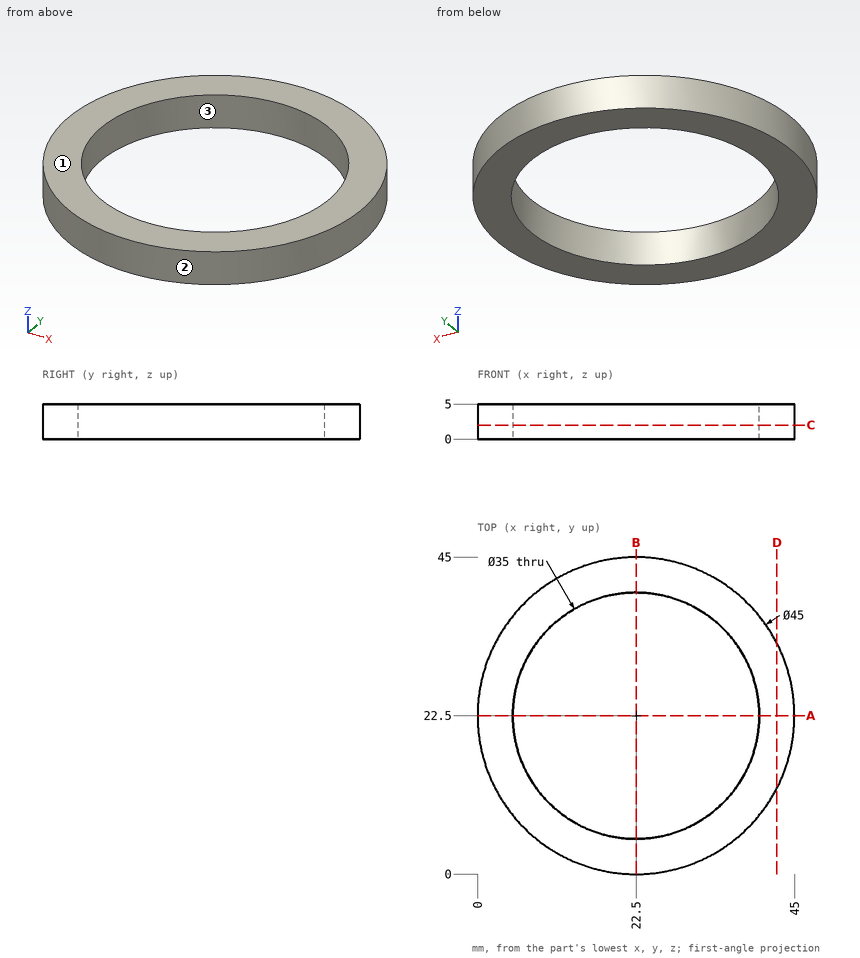
Print and shaded views of the part. All mm, measured from the part's lowest x, y and z. Round coordinates to 2 decimals unless told otherwise and drop trailing zeros. Write each loop counter-clockwise with the first axis right and the second up, starting at its lowest first coordinate (ties: lowest second). Pieces come first, ordered by that corner, then holes. Notation, with made-up numbers: (-29, 76) - (-11, 76) arc R33 ccw to (-11, 113) - close; hole circle Ø10 at (-28, 36). An arc over 180 degrees is marked (long way). One line per question, with ' | ' between items.
1. Drop flat-ended pins along their axis: pin 1 Ø2 at (y, z) = (31.5, 1) entering from -X; pin 2 Ø1.5 at (y, z) = (19.5, 2) entering from -X; pin 3 Ø2 at (x, z) = (13, 3.5) entering from -Y. Give the stop position or say it passes through.
Results are:
pin 1: x = 1.47 | pin 2: x = 0.11 | pin 3: y = 1.67
2. Mould opens along X. For the marked faces 1, 2 and 3 say: released by +X, released by -X, zero draft, split by the parting line, or undercut.
Results are:
face 1: zero draft | face 2: split by the parting line | face 3: undercut
3. Band-saw the part on C-C, the plane z = 2. Write the cut outline in (x, y), and give its area (3 significant figures).
Results are:
outline: circle Ø45 at (22.5, 22.5); hole circle Ø35 at (22.5, 22.5) | area: 628 mm^2
4. Drill centre lines: line 1 along Y through (x, z) = (22.5, 1.2); line 2 along Y through (x, z) = (10, 3.4); line 3 along X through (y, z) = (34.5, 2.5). Where is each one in solid material? Low to high. Write a range as from..to.
Results are:
line 1: 0..5, 40..45 | line 2: 3.79..10.25, 34.75..41.21 | line 3: 3.47..9.76, 35.24..41.53
5. Band-saw the part on A-A, the plane y = 22.5. Write the cut outline in (x, z).
Results are:
outline: (0, 0) - (5, 0) - (5, 5) - (0, 5) - close; (40, 0) - (45, 0) - (45, 5) - (40, 5) - close
6. Band-saw the part on D-D, the plane x = 42.5. Write the cut outline in (y, z), and give its area (3 significant figures).
Results are:
outline: (12.19, 0) - (32.81, 0) - (32.81, 5) - (12.19, 5) - close | area: 103 mm^2
